Check sheet for the drawn part. Datum: minimum x, y, z corner. Units: mm. A direction names the side the tool comes from. Give positions to 0.01 mm unless a question says otherwise; leave off trailing zeros. Write each loop counter-clockwise with the first axis right and the second up, starting at its lowest first coordinate (ties: lowest second). Pieces come first, ordered by that corner, then holes. Notation, with made-up numbers: (32, 32) -> (58, 32) arc R9 ccw to (58, 44) -> close; hole circle Ø2 at (14.25, 74.25). An arc over 180 degrees is marked (long way). Answer as CSV lines item,"result". Start each with the question number.
1) Sectioned sample at B-B on z = 4. Record the cut outline in (x, y), and give its area (3 significant figures).
2) Sectioned sample at C-C on y = 12. Record the cut outline in (x, z).
3) Tool access check on the marked faces 1, 2 and 3. Record the directions out of +Z, -Z, +X, -X, +Y, -Y that give a thin tool (end or side, any length) a straight path to the whole face; none if there is none.
4) Sectioned sample at A-A on x = 4. Record the cut outline in (y, z).
5) Material ranges on L1, parallel to X at y = 20.5, z = 4.25; L2, parallel to X at y = 6.5, z = 0.5, recorded low to high.
6) Gauge pin test, flat ends, axial feed: pin 1 Ø2 at (x, y) = (4.5, 27) entering from +Z; pin 2 Ø2 at (y, z) = (35.5, 4.5) entering from +X. Record the tip position at first contact, or that the pin passes through.
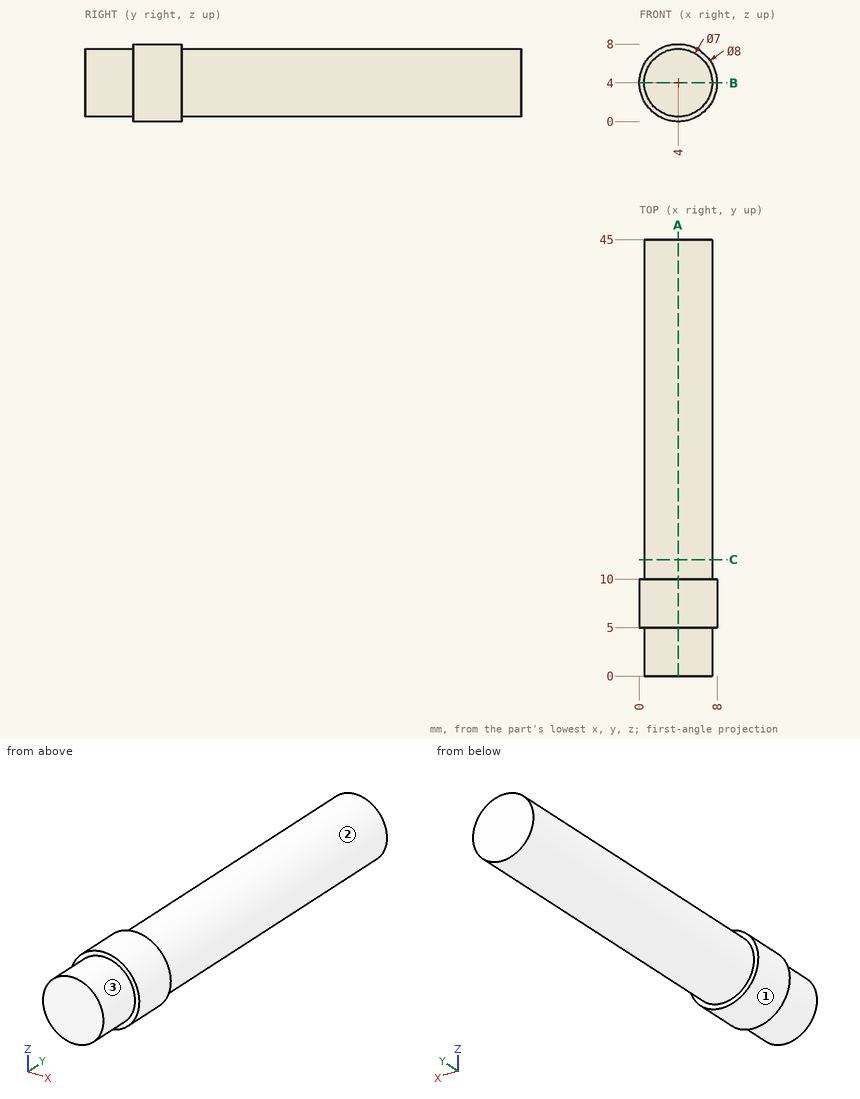
Ans:
1,outline,"(0, 5) -> (0.5, 5) -> (0.5, 0) -> (7.5, 0) -> (7.5, 5) -> (8, 5) -> (8, 10) -> (7.5, 10) -> (7.5, 45) -> (0.5, 45) -> (0.5, 10) -> (0, 10) -> close"
1,area,"320 mm²"
2,outline,"circle Ø7 at (4, 4)"
3,face 1,"+Y, -Y"
3,face 2,"+Y"
3,face 3,"-Y"
4,outline,"(0, 0.5) -> (5, 0.5) -> (5, 0) -> (10, 0) -> (10, 0.5) -> (45, 0.5) -> (45, 7.5) -> (10, 7.5) -> (10, 8) -> (5, 8) -> (5, 7.5) -> (0, 7.5) -> close"
5,L1,"x = 0.51 to 7.49"
5,L2,"x = 2.06 to 5.94"
6,pin 1,"stops at z = 7.5"
6,pin 2,"stops at x = 7.5"
